Could you check a few things on this model? Use its own coordinates, in mm. Face numbers are marked on the shaded views. A direction names the side the tool comes from. Give positions to 0.01 mm unless a question says otherwise; leave off trailing zeros. Write each loop counter-clockwise with the first axis right and the second up, starting at its lowest first coordinate (ties: lowest second). Pieces come first, ordered by that corner, then holes. Notation, with made-up numbers: (67, 26.25) - (87, 26.25) arc R19 cw to (87, 57.25) - close; hole circle Ø11 at (9, 88.25). An arc over 180 degrees is marked (long way). Answer in a Markdown table with one row per item.
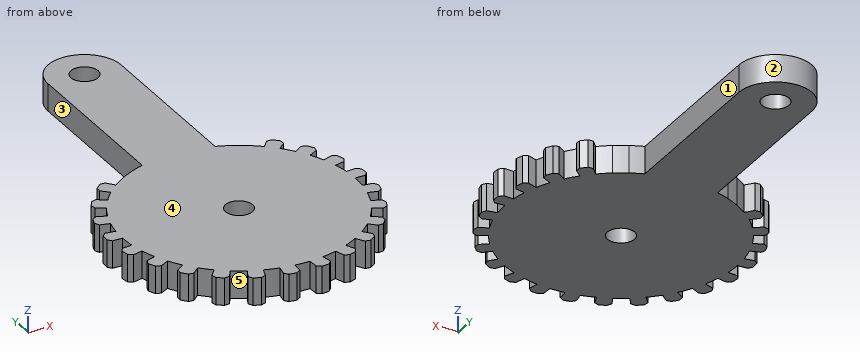
from build123d import *

# Parameters (mm, degrees)
SKETCH1_R           = 1.5
BOSS_EXTRUDE2_DEPTH = 3


with BuildPart() as part:
    # Sketch1 → Boss-Extrude2 (new body)
    with BuildSketch(Plane.XY):
        with BuildLine():
            Line((-4, 31), (-4, 12.106300013))
            ThreePointArc((-4, 12.106300013), (-4.733275563, 11.838859846), (-5.448812758, 11.527052508))
            ThreePointArc((-5.448812758, 11.527052508), (-6.142359345, 11.172910171), (-6.812992455, 10.777088374))
            ThreePointArc((-6.812992455, 10.777088374), (-7.494261967, 10.314966678), (-8.144289673, 9.809844327))
            Line((-8.144289673, 9.809844327), (-8.862903468, 10.675418826))
            Line((-8.862903468, 10.675418826), (-9.445525531, 10.669796035))
            Line((-9.445525531, 10.669796035), (-10.055652175, 10.096848981))
            Line((-10.055652175, 10.096848981), (-10.097847012, 9.515729647))
            Line((-10.097847012, 9.515729647), (-9.27910266, 8.744184))
            ThreePointArc((-9.27910266, 8.744184), (-9.824043845, 8.127155869), (-10.328030916, 7.476247548))
            Line((-10.328030916, 7.476247548), (-11.239327761, 8.13591645))
            Line((-11.239327761, 8.13591645), (-11.80224735, 7.985578094))
            Line((-11.80224735, 7.985578094), (-12.250719604, 7.278898898))
            Line((-12.250719604, 7.278898898), (-12.147070312, 6.705543068))
            Line((-12.147070312, 6.705543068), (-11.162172719, 6.161850387))
            ThreePointArc((-11.162172719, 6.161850387), (-11.536544919, 5.428685967), (-11.862823992, 4.672890641))
            Line((-11.862823992, 4.672890641), (-12.909543756, 5.085204521))
            Line((-12.909543756, 5.085204521), (-13.417390562, 4.799596912))
            Line((-13.417390562, 4.799596912), (-13.676029266, 4.003588828))
            Line((-13.676029266, 4.003588828), (-13.43304851, 3.474022556))
            Line((-13.43304851, 3.474022556), (-12.343882415, 3.192345052))
            ThreePointArc((-12.343882415, 3.192345052), (-12.524162447, 2.389111761), (-12.652232208, 1.575918828))
            Line((-12.652232208, 1.575918828), (-13.768605638, 1.71497049))
            Line((-13.768605638, 1.71497049), (-14.189469779, 1.312039404))
            Line((-14.189469779, 1.312039404), (-14.242023712, 0.476718548))
            Line((-14.242023712, 0.476718548), (-13.874978867, 0.024216431))
            Line((-13.874978867, 0.024216431), (-12.749980581, 0.022252937))
            ThreePointArc((-12.749980581, 0.022252937), (-12.724840787, -0.800579124), (-12.646654143, -1.62007376))
            Line((-12.646654143, -1.62007376), (-13.762535391, -1.763021444))
            Line((-13.762535391, -1.763021444), (-14.069972424, -2.257958364))
            Line((-14.069972424, -2.257958364), (-13.91313943, -3.080105712))
            Line((-13.91313943, -3.080105712), (-13.445093273, -3.427111302))
            Line((-13.445093273, -3.427111302), (-12.354950575, -3.149237412))
            ThreePointArc((-12.354950575, -3.149237412), (-12.125970583, -3.939966678), (-11.846440287, -4.714271155))
            Line((-11.846440287, -4.714271155), (-12.89171443, -5.130236257))
            Line((-12.89171443, -5.130236257), (-13.066406957, -5.686080305))
            Line((-13.066406957, -5.686080305), (-12.710041429, -6.443395602))
            Line((-12.710041429, -6.443395602), (-12.170403021, -6.663101027))
            Line((-12.170403021, -6.663101027), (-11.183613587, -6.122849592))
            ThreePointArc((-11.183613587, -6.122849592), (-10.76518105, -6.831791636), (-10.30187102, -7.512253556))
            Line((-10.30187102, -7.512253556), (-11.210859639, -8.175099458))
            Line((-11.210859639, -8.175099458), (-11.241831085, -8.756924908))
            Line((-11.241831085, -8.756924908), (-10.70832478, -9.401823249))
            Line((-10.70832478, -9.401823249), (-10.131001588, -9.48042361))
            Line((-10.131001588, -9.48042361), (-9.309569027, -8.711740614))
            ThreePointArc((-9.309569027, -8.711740614), (-8.727975601, -9.29435), (-8.109997309, -9.838213438))
            Line((-8.109997309, -9.838213438), (-8.825585306, -10.706291095))
            Line((-8.825585306, -10.706291095), (-8.710889622, -11.277539713))
            Line((-8.710889622, -11.277539713), (-8.033764703, -11.769499764))
            Line((-8.033764703, -11.769499764), (-7.455032066, -11.702056311))
            Line((-7.455032066, -11.702056311), (-6.850570006, -10.753240934))
            ThreePointArc((-6.850570006, -10.753240934), (-6.142359345, -11.172910171), (-5.40854264, -11.546002187))
            Line((-5.40854264, -11.546002187), (-5.885766991, -12.564767086))
            Line((-5.885766991, -12.564767086), (-5.632610928, -13.089545223))
            Line((-5.632610928, -13.089545223), (-4.854413643, -13.397655324))
            Line((-4.854413643, -13.397655324), (-4.310635461, -13.188405776))
            Line((-4.310635461, -13.188405776), (-3.961124478, -12.119075578))
            ThreePointArc((-3.961124478, -12.119075578), (-3.170796061, -12.349435304), (-2.367249346, -12.528313156))
            Line((-2.367249346, -12.528313156), (-2.576124288, -13.633752552))
            Line((-2.576124288, -13.633752552), (-2.200414573, -14.079086466))
            Line((-2.200414573, -14.079086466), (-1.370041921, -14.183986927))
            Line((-1.370041921, -14.183986927), (-0.895385777, -13.846079204))
            Line((-0.895385777, -13.846079204), (-0.82278693, -12.723424133))
            ThreePointArc((-0.82278693, -12.723424133), (0, -12.75), (0.82278693, -12.723424133))
            Line((0.82278693, -12.723424133), (0.895385777, -13.846079204))
            Line((0.895385777, -13.846079204), (1.370041921, -14.183986927))
            Line((1.370041921, -14.183986927), (2.200414573, -14.079086466))
            Line((2.200414573, -14.079086466), (2.576124288, -13.633752552))
            Line((2.576124288, -13.633752552), (2.367249346, -12.528313156))
            ThreePointArc((2.367249346, -12.528313156), (3.170796061, -12.349435304), (3.961124478, -12.119075578))
            Line((3.961124478, -12.119075578), (4.310635461, -13.188405776))
            Line((4.310635461, -13.188405776), (4.854413643, -13.397655324))
            Line((4.854413643, -13.397655324), (5.632610928, -13.089545223))
            Line((5.632610928, -13.089545223), (5.885766991, -12.564767086))
            Line((5.885766991, -12.564767086), (5.40854264, -11.546002187))
            ThreePointArc((5.40854264, -11.546002187), (6.142359345, -11.172910171), (6.850570006, -10.753240934))
            Line((6.850570006, -10.753240934), (7.455032066, -11.702056311))
            Line((7.455032066, -11.702056311), (8.033764703, -11.769499764))
            Line((8.033764703, -11.769499764), (8.710889622, -11.277539713))
            Line((8.710889622, -11.277539713), (8.825585306, -10.706291095))
            Line((8.825585306, -10.706291095), (8.109997309, -9.838213438))
            ThreePointArc((8.109997309, -9.838213438), (8.727975601, -9.29435), (9.309569027, -8.711740614))
            Line((9.309569027, -8.711740614), (10.131001588, -9.48042361))
            Line((10.131001588, -9.48042361), (10.70832478, -9.401823249))
            Line((10.70832478, -9.401823249), (11.241831085, -8.756924908))
            Line((11.241831085, -8.756924908), (11.210859639, -8.175099458))
            Line((11.210859639, -8.175099458), (10.30187102, -7.512253556))
            ThreePointArc((10.30187102, -7.512253556), (10.76518105, -6.831791636), (11.183613587, -6.122849592))
            Line((11.183613587, -6.122849592), (12.170403021, -6.663101027))
            Line((12.170403021, -6.663101027), (12.710041429, -6.443395602))
            Line((12.710041429, -6.443395602), (13.066406957, -5.686080305))
            Line((13.066406957, -5.686080305), (12.89171443, -5.130236257))
            Line((12.89171443, -5.130236257), (11.846440287, -4.714271155))
            ThreePointArc((11.846440287, -4.714271155), (12.125970583, -3.939966678), (12.354950575, -3.149237412))
            Line((12.354950575, -3.149237412), (13.445093273, -3.427111302))
            Line((13.445093273, -3.427111302), (13.91313943, -3.080105712))
            Line((13.91313943, -3.080105712), (14.069972424, -2.257958364))
            Line((14.069972424, -2.257958364), (13.762535391, -1.763021444))
            Line((13.762535391, -1.763021444), (12.646654143, -1.62007376))
            ThreePointArc((12.646654143, -1.62007376), (12.724840787, -0.800579124), (12.749980581, 0.022252937))
            Line((12.749980581, 0.022252937), (13.874978867, 0.024216431))
            Line((13.874978867, 0.024216431), (14.242023712, 0.476718548))
            Line((14.242023712, 0.476718548), (14.189469779, 1.312039404))
            Line((14.189469779, 1.312039404), (13.768605638, 1.71497049))
            Line((13.768605638, 1.71497049), (12.652232208, 1.575918828))
            ThreePointArc((12.652232208, 1.575918828), (12.524162447, 2.389111761), (12.343882415, 3.192345052))
            Line((12.343882415, 3.192345052), (13.43304851, 3.474022556))
            Line((13.43304851, 3.474022556), (13.676029266, 4.003588828))
            Line((13.676029266, 4.003588828), (13.417390562, 4.799596912))
            Line((13.417390562, 4.799596912), (12.909543756, 5.085204521))
            Line((12.909543756, 5.085204521), (11.862823992, 4.672890641))
            ThreePointArc((11.862823992, 4.672890641), (11.536544919, 5.428685967), (11.162172719, 6.161850387))
            Line((11.162172719, 6.161850387), (12.147070312, 6.705543068))
            Line((12.147070312, 6.705543068), (12.250719604, 7.278898898))
            Line((12.250719604, 7.278898898), (11.80224735, 7.985578094))
            Line((11.80224735, 7.985578094), (11.239327761, 8.13591645))
            Line((11.239327761, 8.13591645), (10.328030916, 7.476247548))
            ThreePointArc((10.328030916, 7.476247548), (9.824043845, 8.127155869), (9.27910266, 8.744184))
            Line((9.27910266, 8.744184), (10.097847012, 9.515729647))
            Line((10.097847012, 9.515729647), (10.055652175, 10.096848981))
            Line((10.055652175, 10.096848981), (9.445525531, 10.669796035))
            Line((9.445525531, 10.669796035), (8.862903468, 10.675418826))
            Line((8.862903468, 10.675418826), (8.144289673, 9.809844327))
            ThreePointArc((8.144289673, 9.809844327), (7.494261967, 10.314966678), (6.812992455, 10.777088374))
            ThreePointArc((6.812992455, 10.777088374), (6.142359345, 11.172910171), (5.448812758, 11.527052508))
            ThreePointArc((5.448812758, 11.527052508), (4.733275563, 11.838859846), (4, 12.106300013))
            Line((4, 12.106300013), (4, 31))
            ThreePointArc((4, 31), (0, 35), (-4, 31))
        make_face()
        Circle(SKETCH1_R, mode=Mode.SUBTRACT)
        with Locations((0, 31)):
            Circle(SKETCH1_R, mode=Mode.SUBTRACT)
    extrude(amount=BOSS_EXTRUDE2_DEPTH)


solid = part.part
1) Imagine slicing it at B-B (z = 2.1). State how many separate pieces and enclosed holes the cut face has, then the cut area to 3 significant figures.
Check values:
| item | result |
|---|---|
| separate pieces | 1 |
| enclosed holes | 2 |
| area | 715 mm2 |
2) If I drill on line 1 (Y direction, x = 0, z = 2.45); line 2 (X direction, y = 10, z = 2.15); line 3 (X direction, y = -6.5, z = 1), over which ranges is the centre line in solid material (lowest first)?
Check values:
| item | result |
|---|---|
| line 1 | y = -12.75 to -1.5, 1.5 to 29.5, 32.5 to 35 |
| line 2 | x = -10.06 to -8.3, -7.91 to 7.91, 8.3 to 10.06 |
| line 3 | x = -12.57 to -11.87, -10.97 to 10.97, 11.87 to 12.57 |
3) Imagine slicing it at C-C (y = 26). List the corners of the cut face in (x, z) for me.
Check values:
| item | result |
|---|---|
| outline | (-4, 0) - (4, 0) - (4, 3) - (-4, 3) - close |
4) We'd pull the mould along X, two halves only. Please class the marked faces 3, 4 and 5: +X half, -X half, draft (parallel to the pull), parting line (faces both ways), or undercut.
Check values:
| item | result |
|---|---|
| face 3 | -X half |
| face 4 | draft |
| face 5 | undercut |
5) On a 3-axis mill with a long thin cutter (end or side, diameter ignored), from which of +Z, -Z, +X, -X, +Y, -Y can I reach the whole of each face in a straight line? I mean the marked faces 1 and 2. Say none if no direction works.
Check values:
| item | result |
|---|---|
| face 1 | +Z, -Z, +X, +Y |
| face 2 | +Z, -Z, +Y |
6) Will these pins go through, and if not, where does the flat tip stop? P1, Ø0.9, axis at y = 26, z = 2, coming from the -X side; P2, Ø10, axis at x = -8, y = 21, coming from the +Z side.
Check values:
| item | result |
|---|---|
| P1 | stops at x = -4 |
| P2 | stops at z = 3 |
7) Imagine slicing it at A-A (x = 0). List the corners of the cut face in (y, z) for me, then the cut area to 3 significant figures.
Check values:
| item | result |
|---|---|
| outline | (-12.75, 0) - (-1.5, 0) - (-1.5, 3) - (-12.75, 3) - close; (1.5, 0) - (29.5, 0) - (29.5, 3) - (1.5, 3) - close; (32.5, 0) - (35, 0) - (35, 3) - (32.5, 3) - close |
| area | 125 mm2 |
